Input: part model. Units: mm. Frame: model coordinates. Face numbers are marked on the shaded views. A direction names the side the tool comes from. Give positions to 0.01 mm unless a question says otherwise; leave off trailing zeros. Loops run counter-clockwise (first coordinate to the right, second up) from the corner with the lowest first, then second, coordinate; pieces in that order, holes last. Notation, with made-up numbers: (2.25, 5) -> (35.25, 5) arc R8 cw to (35.25, 17) -> close; hole circle Ø3 at (-5, 49.5). An arc over 180 degrees is marked (long way). Answer as a JSON object with one key per item and string values.
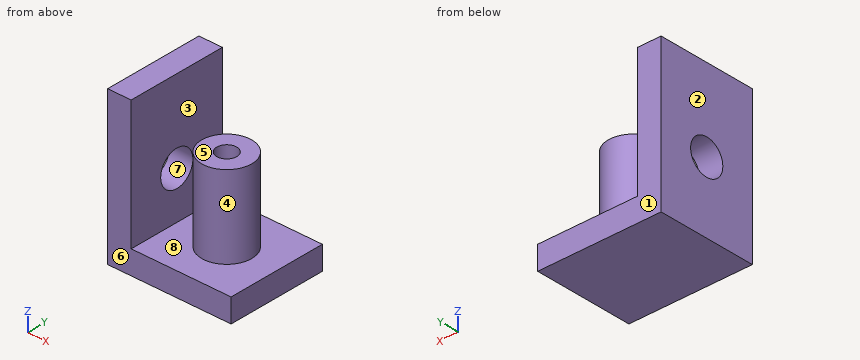
```python
from build123d import *

# Parameters (mm, degrees)
SKETCH007_W   = 8.5
SKETCH007_H   = 8.5
PAD005_DEPTH  = 2
SKETCH008_R   = 2.125
SKETCH008_R_2 = 0.85
PAD006_DEPTH  = 7
SKETCH009_W   = 8.5
SKETCH009_H   = 13
SKETCH009_R   = 1.5
PAD007_DEPTH  = 2


with BuildPart() as part:
    # Sketch007 → Pad005 (new body)
    with BuildSketch(Plane.XY):
        with Locations((4.25, 4.25)):
            Rectangle(SKETCH007_W, SKETCH007_H)
    extrude(amount=PAD005_DEPTH)

    # Sketch008 (on Face6 of Pad005) → Pad006 (join)
    with BuildSketch(Plane.XY.offset(2)):
        with Locations((4.25, 4.25)):
            Circle(SKETCH008_R)
        with Locations((4.25, 4.25)):
            Circle(SKETCH008_R_2, mode=Mode.SUBTRACT)
    extrude(amount=PAD006_DEPTH)

    # Sketch009 (on Face2 of Pad006) → Pad007 (join)
    with BuildSketch(Plane(origin=(0, 0, 0), x_dir=(0, -1, 0), z_dir=(-1, 0, 0))):
        with Locations((-4.25, 6.5)):
            Rectangle(SKETCH009_W, SKETCH009_H)
        with Locations((-4.25, 6)):
            Circle(SKETCH009_R, mode=Mode.SUBTRACT)
    extrude(amount=PAD007_DEPTH)


solid = part.part
```
Q1. Ray query, line 1 along Y through (x, z) = (4.25, 4.5) (3 decimals); line 2 along Z through (x, y) = (-1.35, 4.25); line 3 along X through (y, z) = (2.25, 11). Return the intervals inside material, ascending.
Evaluation:
{"line 1": "y = 2.125 to 3.4, 5.1 to 6.375", "line 2": "z = 0 to 4.5, 7.5 to 13", "line 3": "x = -2 to 0"}
Q2. Access query for the marked faces 5, 6, 7 and 8. Directions: +Z, -Z, +X, -X, +Y, -Y. A direction counts if a zero-diameter tool reaches every point of the face in a straight line with its end or side. Return the directions, or none.
Evaluation:
{"face 5": "+Z, +X, +Y, -Y", "face 6": "+Z, -Z, +X, -X, -Y", "face 7": "-X", "face 8": "+Z"}
Q3. Draft query along X for the marked faces 1, 2, 3 and 4. Return one class per face: +X half, -X half, draft (parallel to the pull), parting line (faces both ways), or undercut.
Evaluation:
{"face 1": "draft", "face 2": "-X half", "face 3": "undercut", "face 4": "undercut"}
Q4. Section D-D, the plane y = 7.25. Return the cut outline in (x, z).
Evaluation:
{"outline": "(-2, 0) -> (8.5, 0) -> (8.5, 2) -> (0, 2) -> (0, 13) -> (-2, 13) -> close"}
Q5. Section A-A, the plane y = 4.25. Return the cut outline in (x, z) (3 decimals).
Evaluation:
{"outline": "(-2, 0) -> (8.5, 0) -> (8.5, 2) -> (6.375, 2) -> (6.375, 9) -> (5.1, 9) -> (5.1, 2) -> (3.4, 2) -> (3.4, 9) -> (2.125, 9) -> (2.125, 2) -> (0, 2) -> (0, 4.5) -> (-2, 4.5) -> close; (-2, 7.5) -> (0, 7.5) -> (0, 13) -> (-2, 13) -> close"}
Q6. Section C-C, the plane x = -1. Return the cut outline in (y, z).
Evaluation:
{"outline": "(0, 0) -> (8.5, 0) -> (8.5, 13) -> (0, 13) -> close; hole circle Ø3 at (4.25, 6)"}
Q7. Section B-B, the plane z = 6. Return the cut outline in (x, y) (3 decimals).
Evaluation:
{"outline": "(-2, 0) -> (0, 0) -> (0, 2.75) -> (-2, 2.75) -> close; (-2, 5.75) -> (0, 5.75) -> (0, 8.5) -> (-2, 8.5) -> close; circle Ø4.25 at (4.25, 4.25); hole circle Ø1.7 at (4.25, 4.25)"}
Q8. Pin query (flat end, axial travel): pin 1 (0.8 mm diameter, centred on x = 4.5, y = 4, fed in from +Z); pin 2 (2 mm diameter, centred on y = 4.5, z = 10.5, fed in from +X); pin 3 (2.5 mm diameter, centred on y = 6, z = 8, fed in from +X). Return the tip coordinate at first contact, or that it passes through.
Evaluation:
{"pin 1": "stops at z = 2", "pin 2": "stops at x = 0", "pin 3": "stops at x = 6.32"}
